```python
from build123d import *

# Parameters (mm, degrees)
F1_DEPTH = 5
F3_D     = 3.2
F5_DEPTH = 30


with BuildPart() as f1:
    # F0 (on Top) → F1 (new body)
    with BuildSketch(Plane.XY):
        Polygon((0, 20), (0, 0), (40, 0), (40, -40), (60, -40), (60, 20), align=None)
    extrude(amount=F1_DEPTH)

    # F3 (through all)
    with Locations(Plane.XY.offset(5)):
        with Locations((15, 10), (50, -25)):
            Hole(F3_D / 2)

    # F4 (on face) → F5 (join)
    with BuildSketch(Plane.XY.offset(5)):
        with BuildLine():
            ThreePointArc((40, -20), (54.1421356237, -14.1421356237), (60, 0))
            ThreePointArc((60, 0), (54.1421356237, 14.1421356237), (40, 20))
            ThreePointArc((40, 20), (25.8578643763, 14.1421356237), (20, 0))
            Line((20, 0), (40, 0))
            Line((40, 0), (40, -20))
        make_face()
        with BuildLine():
            ThreePointArc((20, 0), (25.8578643763, -14.1421356237), (40, -20))
            Line((40, -20), (40, 0))
            Line((40, 0), (20, 0))
        make_face()
    extrude(amount=-F5_DEPTH)


solid = f1.part
```
Work out the finished part from the listing and answer in its coordinate system (mm). A direction names the side the tool comes from. Give positions to 0.01 mm unless a question says otherwise; leave off trailing zeros. Loops run counter-clockwise (first coordinate to the right, second up) from the corner with the lowest first, then second, coordinate; pieces in that order, holes last. Notation, with made-up numbers: M -0.75,73 L 35.25,73 A16 ccw 35.25,83 Z; hole C 0.25,9.5 d8. An arc over 180 degrees is marked long. One line per item, written item: value. Start each with the question number.
1. Find section B-B (y = -25). Give the vertices of the cut face in (x, z).
2. Find section A-A (x = 15). Give the vertices of the cut face in (y, z).
3. Find section C-C (x = 56). Give the vertices of the cut face in (y, z), and give its area (3 significant figures).
4. Determine the mould class of faces 5 (the face through (0, 10, 2)), 6 (the face through (48.474, -24.519, 2.465)), 7 (the face through (11, 10, 0)), 8 (the face through (16.6, 10.07, 2.47)) for opening direction X: released by +X, released by -X, zero draft, split by the parting line, or undercut.
5. Find section D-D (y = -4). Give the vertices of the cut face in (x, z), and give its area (3 significant figures).
6. Find the intervals of material crossed by probe 1 along Y at (x, z) = (50, 3.4); probe 2 along Y at (x, z) = (15, 3.95); probe 3 along Z at (x, y) = (10, 8.5), in increasing order.
7. Which of the six approach directions +Z, -Z, +X, -X, +Y, -Y give full straight-line access (tool end or side, diameter ignored) to faces 1 (the face through (10, 0, 2)), 2 (the face through (36, -3, 5)), 3 (the face through (55, 16, 0)), 4 (the face through (50, -29, 0))?
8. Each of these flat-tipped pins is pushed along its axis until it touches: P1, Ø8, axis at y = -11.5, z = -2.5, coming from the -X side; P2, Ø2.5, axis at x = 12.5, z = 1.5, coming from the -Y side; P3, Ø1, axis at y = -6, z = -10, coming from the -X side. Where does it stop, or does it pass through?
Reported:
1. outline: M 40,0 L 48.4,0 L 48.4,5 L 40,5 Z; M 51.6,0 L 60,0 L 60,5 L 51.6,5 Z
2. outline: M 0,0 L 8.4,0 L 8.4,5 L 0,5 Z; M 11.6,0 L 20,0 L 20,5 L 11.6,5 Z
3. outline: M -40,0 L -12,0 L -12,-25 L 12,-25 L 12,0 L 20,0 L 20,5 L -40,5 Z
3. area: 900 mm²
4. face 5: released by -X
4. face 6: undercut
4. face 7: zero draft
4. face 8: undercut
5. outline: M 20.4,-25 L 59.6,-25 L 59.6,0 L 60,0 L 60,5 L 20.4,5 Z
5. area: 1,180 mm²
6. probe 1: y = -40 to -26.6, -23.4 to 20
6. probe 2: y = 0 to 8.4, 11.6 to 20
6. probe 3: z = 0 to 5
7. face 1: +Z, -Z, -X, -Y
7. face 2: +Z, +X, -X, +Y, -Y
7. face 3: -Z, +X, +Y
7. face 4: -Z, +X, -Y
8. P1: stops at x = 21.46
8. P2: stops at y = 0
8. P3: stops at x = 20.77
